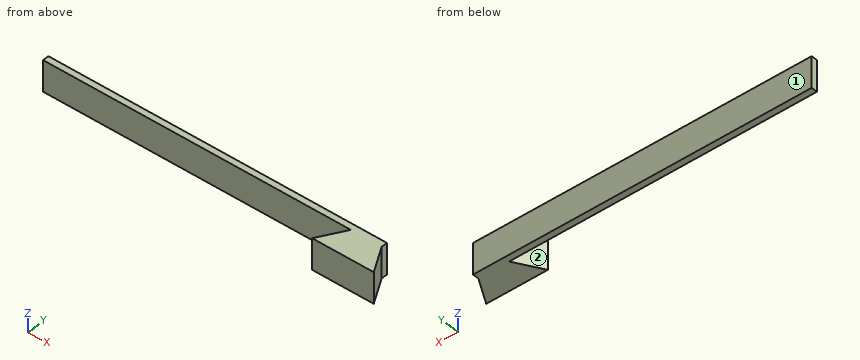
```python
from build123d import *

# Parameters (mm, degrees)
SALIENTE_EXTRUIR1_DEPTH = 100
CROQUIS2_W              = 100
CROQUIS2_H              = 100
SALIENTE_EXTRUIR2_DEPTH = 20
CROQUIS3_W              = 100
CROQUIS3_H              = 20
SALIENTE_EXTRUIR3_DEPTH = 1000


with BuildPart() as part:
    # Croquis1 → Saliente-Extruir1 (new body)
    with BuildSketch(Plane.XY):
        Polygon((0, 0), (50, 86.602540378), (150, 86.602540378), (200, 0), align=None)
    extrude(amount=SALIENTE_EXTRUIR1_DEPTH)

    # Croquis2 → Saliente-Extruir2 (add)
    with BuildSketch(Plane(origin=(0, 86.602540378, 0), x_dir=(1, 0, 0), z_dir=(0, 1, 0))):
        with Locations((100, -50)):
            Rectangle(CROQUIS2_W, CROQUIS2_H)
    extrude(amount=SALIENTE_EXTRUIR2_DEPTH)

    # Croquis3 → Saliente-Extruir3 (add)
    with BuildSketch(Plane.ZY.offset(-50)):
        with Locations((50, 96.602540378)):
            Rectangle(CROQUIS3_W, CROQUIS3_H)
    extrude(amount=SALIENTE_EXTRUIR3_DEPTH)


solid = part.part
```
Here's how the part is built. I have some questions about the finished solid (model axes, mm). Face numbers are marked on the shaded views. A direction names the side the tool comes from. Round coordinates to 2 decimals unless told otherwise and drop trailing zeros. Order: outer loops, then holes, each group sorted by start corner. A loop starts at its lowest first (then second) coordinate and runs counter-clockwise, first axis right, second up. Notation, with made-up numbers: (48.5, 31) -> (85.5, 31) arc R36 cw to (85.5, 69) -> close; hole circle Ø8 at (84.25, 29). An arc over 180 degrees is marked (long way). Use a Markdown table: item, result. Add a question column.
(1) Suppose I cut it at A-A, the plane z = 78. Please give me the cut outline in (x, y), and give its area (3 significant figures).
(2) Suppose I cut it at D-D, the plane y = 61. Please give me the cut outline in (x, z).
(3) For the marked faces 1 and 2, which set-ups out of +Z, -Z, +X, -X, +Y, -Y let a thin tool reach every point of the face, with its end or its side?
(4) Suppose I cut it at B-B, the plane x = 36. Please give me the cut outline in (y, z), and give its area (3 significant figures).
(5) I need wall thicknesses on line 1 along X through (y, z) = (100.5, 88); line 2 along Y through (x, z) = (-622, 93); line 3 along Y through (x, z) = (15.5, 11). Which ranges of each line are inside material? Lowest first, please.
(6) Suppose I cut it at C-C, the plane x = -79. Please give me the cut outline in (y, z).
(7) For pin 1 Ø6 at (y, z) = (97, 53.5) entering from +X; pin 2 Ø5 at (x, z) = (-267.5, 74) entering from -Y; pin 3 Ø10 at (y, z) = (71, 81) entering from +X, each with a flat end and sliding along its axis, tell me the tip position at first contact or that it passes through.
Verdict:
| question | item | result |
|---|---|---|
| 1 | outline | (-950, 86.6) -> (50, 86.6) -> (0, 0) -> (200, 0) -> (150, 86.6) -> (150, 106.6) -> (-950, 106.6) -> close |
| 1 | area | 35,000 mm2 |
| 2 | outline | (35.22, 0) -> (164.78, 0) -> (164.78, 100) -> (35.22, 100) -> close |
| 3 | face 1 | +Z, -Z, +X, -X, +Y |
| 3 | face 2 | +Z, -Z, -X |
| 4 | outline | (0, 0) -> (62.35, 0) -> (62.35, 100) -> (0, 100) -> close; (86.6, 0) -> (106.6, 0) -> (106.6, 100) -> (86.6, 100) -> close |
| 4 | area | 8,240 mm2 |
| 5 | line 1 | -950 to 150 |
| 5 | line 2 | 86.6 to 106.6 |
| 5 | line 3 | 0 to 26.85, 86.6 to 106.6 |
| 6 | outline | (86.6, 0) -> (106.6, 0) -> (106.6, 100) -> (86.6, 100) -> close |
| 7 | pin 1 | x = 150 |
| 7 | pin 2 | y = 86.6 |
| 7 | pin 3 | x = 161.89 |
